from build123d import *

# Parameters (mm, degrees)
SKETCH1_W           = 21
SKETCH1_H           = 15
BOSS_EXTRUDE1_DEPTH = 20
SKETCH2_R           = 4.95
BOSS_EXTRUDE2_DEPTH = 9
CHAMFER1_SIZE       = 1
SKETCH3_R           = 2.2
CUT_EXTRUDE1_DEPTH  = 54.824529308
SKETCH4_R           = 4.25
CUT_EXTRUDE2_DEPTH  = 5


with BuildPart() as part:
    # Sketch1 → Boss-Extrude1 (new body)
    with BuildSketch(Plane(origin=(0, 0, 0), x_dir=(0, 0, -1), z_dir=(1, 0, 0))):
        with Locations((-37.166339855, -9.630048879)):
            Rectangle(SKETCH1_W, SKETCH1_H)
    extrude(amount=BOSS_EXTRUDE1_DEPTH)

    # Sketch2 → Boss-Extrude2 (add)
    with BuildSketch(Plane(origin=(0, 0, 26.666339855), x_dir=(-1, 0, 0), z_dir=(0, 0, -1))):
        with Locations(Location((-10, -9.630048879, 0), (0, 0, 90))):
            Circle(SKETCH2_R)
    extrude(amount=BOSS_EXTRUDE2_DEPTH)

    # Chamfer1
    chamfer1_edges = [part.edges().sort_by_distance(p)[0] for p in [
        (10, -14.580048879, 17.666339855),
    ]]
    chamfer(chamfer1_edges, length=CHAMFER1_SIZE)

    # Sketch3 → Cut-Extrude1 (cut, through all)
    with BuildSketch(Plane(origin=(0, -2.130048879, 0), x_dir=(1, 0, 0), z_dir=(0, 1, 0))):
        with Locations(Location((10, -37.166339855, 0), (0, 0, 270))):
            Circle(SKETCH3_R)
    extrude(amount=-CUT_EXTRUDE1_DEPTH, mode=Mode.SUBTRACT)

    # Sketch4 → Cut-Extrude2 (cut)
    with BuildSketch(Plane(origin=(0, -2.130048879, 0), x_dir=(1, 0, 0), z_dir=(0, 1, 0))):
        with Locations(Location((10, -37.166339855, 0), (0, 0, 270))):
            Circle(SKETCH4_R)
    extrude(amount=-CUT_EXTRUDE2_DEPTH, mode=Mode.SUBTRACT)


solid = part.part
Input: part model. Units: mm. Frame: model coordinates. A direction names the side the tool comes from. Give positions to 0.01 mm unless a question says otherwise; leave off trailing zeros. Write each loop counter-clockwise with the first axis right and the second up, starting at its lowest first coordinate (ties: lowest second). Pieces come first, ordered by that corner, then holes.
Q1. Material intervals for probe 1 along Z at (x, y) = (16.75, -10.25); probe 2 along Y at (x, z) = (8.75, 39.5); probe 3 along Z at (x, y) = (8, -3.5), sorted ascending.
Q2. Section B-B, the plane y = -3.75. Output: boundary loops of the cut face in (x, z), plus the area to 3 significant figures.
Q3. Pull-direction query (Z, two-part tool) for faces 4 (the face through (11.487, -12.06, 35.545)), 5 (the face through (5, -2.13, 37)), 6 (the face through (8, -7.13, 39)), 7 (the face through (10, -10, 47.666)); classes: pulls with the +Z half, pulls with the -Z half, needs draft (parallel to the pull), parting line crosses it, or undercut.
Q4. Set-up query: faces 1 (the face through (6.23, -4.6, 39.13)), 2 (the face through (10, -15, 26.666)), 3 (the face through (7.6, -17.13, 37.3)). Return all of +Z, -Z, +X, -X, +Y, -Y with unobstructed straight access to the full face (end or side cutting, diameter ignored); none if empty.
Q5. First-contact query: P1, Ø8, axis at x = 17, z = 21.5, coming from the -Y side; P2, Ø12, axis at x = 5, z = 25, coming from the +Y side. Flat tips, straight axial feed; report the tip coordinate or a pass-through.
Q6. Section D-D, the plane y = -15.75. Output: boundary loops of the cut face in (x, z), plus the area to 3 significant figures.
Q7. Section A-A, the plane x = 10. Output: boundary loops of the cut face in (y, z), plus the area to 3 significant figures.
Q8. Section C-C, the plane z = 39. Output: boundary loops of the cut face in (x, y).
Filled in:
1. probe 1: z = 26.67 to 47.67
1. probe 2: y = -17.13 to -7.13
1. probe 3: z = 26.67 to 33.42, 40.92 to 47.67
2. outline: (0, 26.67) - (20, 26.67) - (20, 47.67) - (0, 47.67) - close; hole circle Ø8.5 at (10, 37.17)
2. area: 363 mm2
3. face 4: undercut
3. face 5: needs draft
3. face 6: undercut
3. face 7: pulls with the +Z half
4. face 1: +Y
4. face 2: -Z
4. face 3: +Z, -Z, +X, -X, -Y
5. P1: stops at y = -13.57
5. P2: stops at y = -2.13
6. outline: (0, 26.67) - (20, 26.67) - (20, 47.67) - (0, 47.67) - close; hole circle Ø4.4 at (10, 37.17)
6. area: 405 mm2
7. outline: (-17.13, 26.67) - (-14.58, 26.67) - (-14.58, 18.67) - (-13.58, 17.67) - (-5.68, 17.67) - (-4.68, 18.67) - (-4.68, 26.67) - (-2.13, 26.67) - (-2.13, 32.92) - (-7.13, 32.92) - (-7.13, 34.97) - (-17.13, 34.97) - close; (-17.13, 39.37) - (-7.13, 39.37) - (-7.13, 41.42) - (-2.13, 41.42) - (-2.13, 47.67) - (-17.13, 47.67) - close
7. area: 317 mm2
8. outline: (0, -17.13) - (8.78, -17.13) - (8.78, -7.13) - (6.17, -7.13) - (6.17, -2.13) - (0, -2.13) - close; (11.22, -17.13) - (20, -17.13) - (20, -2.13) - (13.83, -2.13) - (13.83, -7.13) - (11.22, -7.13) - close
